Here's how the part is built. I have some questions about the finished solid (model axes, mm). Face numbers are marked on the shaded views. A direction names the side the tool comes from. Give positions to 0.01 mm unless a question says otherwise; leave off trailing zeros. Write each loop counter-clockwise with the first axis right and the second up, starting at its lowest first coordinate (ties: lowest second). Pieces come first, ordered by that corner, then holes. Notation, with made-up numbers: (40.5, 18.25) -> (75.5, 18.25) arc R27 ccw to (75.5, 45.25) -> close; hole circle Ø11 at (-24, -10). An arc over 180 degrees is marked (long way). Use one line per item in the form item = value.
```python
from build123d import *

# Parameters (mm, degrees)
SKETCH_1_W          = 8
SKETCH_1_H          = 48.14748393
SKETCH_1_R          = 1.65
EXTRUDE_1_DEPTH     = 53
EXTRUDE_1_2_DEPTH   = 53
SKETCH_2_W          = 20
SKETCH_2_H          = 3
EXTRUDE_2_DEPTH     = 80
SKETCH_3_R          = 14.5
SKETCH_3_R_2        = 2.25
CUT_EXTRUDE_1_DEPTH = 20
SKETCH_4_W          = 48.14748393
SKETCH_4_H          = 36
CUT_EXTRUDE_2_DEPTH = 15
SKETCH_6_W          = 8
SKETCH_6_H          = 15
CUT_EXTRUDE_4_DEPTH = 6


with BuildPart() as part:
    # Sketch 1 → Extrude 1 (new body)
    with BuildSketch(Plane(origin=(0, 0, 0), x_dir=(1, 0, 0), z_dir=(0, 1, 0))):
        with Locations((44, 0)):
            Rectangle(SKETCH_1_W, SKETCH_1_H)
        with Locations(Location((44, 0, 0), (0, 0, 90))):
            Circle(SKETCH_1_R, mode=Mode.SUBTRACT)
        with Locations(Location((44, -12, 0), (0, 0, 90))):
            Circle(SKETCH_1_R, mode=Mode.SUBTRACT)
        with Locations(Location((44, 12, 0), (0, 0, 270))):
            Circle(SKETCH_1_R, mode=Mode.SUBTRACT)
    extrude(amount=EXTRUDE_1_DEPTH)



with BuildPart() as body_2:
    # Sketch 1 → Extrude 1 2 (new body)
    with BuildSketch(Plane(origin=(0, 0, 0), x_dir=(1, 0, 0), z_dir=(0, 1, 0))):
        with Locations((-44, 0)):
            Rectangle(SKETCH_1_W, SKETCH_1_H)
        with Locations(Location((-44, 0, 0), (0, 0, 270))):
            Circle(SKETCH_1_R, mode=Mode.SUBTRACT)
        with Locations(Location((-44, -12, 0), (0, 0, 270))):
            Circle(SKETCH_1_R, mode=Mode.SUBTRACT)
        with Locations(Location((-44, 12, 0), (0, 0, 90))):
            Circle(SKETCH_1_R, mode=Mode.SUBTRACT)
    extrude(amount=EXTRUDE_1_2_DEPTH)


with BuildPart() as part_1:
    add(part.part)

    add(body_2.part)  # Extrude 2 merges body 2
    # Sketch 2 → Extrude 2 (add)
    with BuildSketch(Plane(origin=(-40, 0, 0), x_dir=(0, 0, -1), z_dir=(1, 0, 0))):
        with Locations((0, 1.5)):
            Rectangle(SKETCH_2_W, SKETCH_2_H)
    extrude(amount=EXTRUDE_2_DEPTH)

    # Sketch 3 → Cut-Extrude 1 (cut)
    with BuildSketch(Plane(origin=(48, 0, 0), x_dir=(0, 0, -1), z_dir=(1, 0, 0))):
        with Locations((-19.073741965, 30)):
            Circle(SKETCH_3_R)
        with Locations((-19.073741965, 47.5)):
            Circle(SKETCH_3_R_2)
        with Locations((-18.617981623, 12.505935792)):
            Circle(SKETCH_3_R_2)
    extrude(amount=-CUT_EXTRUDE_1_DEPTH, mode=Mode.SUBTRACT)

    # Sketch 4 → Cut-Extrude 2 (cut)
    with BuildSketch(Plane.ZY.offset(48)):
        with Locations((0, 35)):
            Rectangle(SKETCH_4_W, SKETCH_4_H)
    extrude(amount=-CUT_EXTRUDE_2_DEPTH, mode=Mode.SUBTRACT)

    # Sketch 6 → Cut-Extrude 4 (cut)
    with BuildSketch(Plane(origin=(0, 17, 0), x_dir=(1, 0, 0), z_dir=(0, 1, 0))):
        with Locations((-44, 0)):
            Rectangle(SKETCH_6_W, SKETCH_6_H)
    extrude(amount=-CUT_EXTRUDE_4_DEPTH, mode=Mode.SUBTRACT)


solid = part_1.part
```
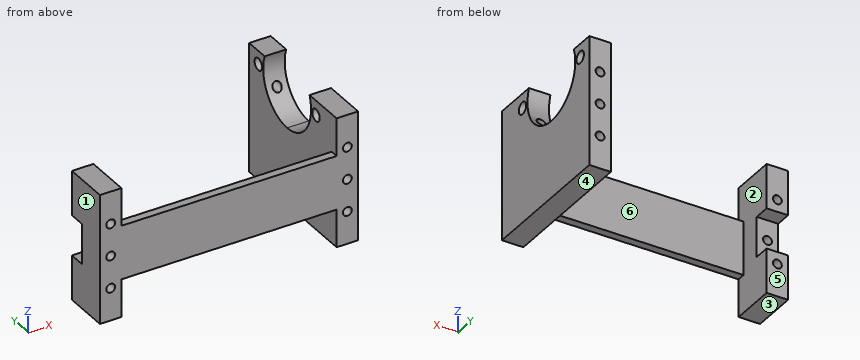
Q1. I want a section at C-C, the plane z = -12. Write out the boundary of the cut face in (x, y).
Result set:
outline = (-48, 0) -> (-45.65, 0) -> (-45.65, 17) -> (-48, 17) -> close; (-42.35, 0) -> (-40, 0) -> (-40, 17) -> (-42.35, 17) -> close; (40, 0) -> (42.35, 0) -> (42.35, 53) -> (40, 53) -> close; (45.65, 0) -> (48, 0) -> (48, 53) -> (45.65, 53) -> close
Q2. If I drill on line 1 along Z through (x, y) = (-44, 7.5); line 2 along X through (y, z) = (7.5, -12); line 3 along X through (y, z) = (3.5, -18), over which ranges is the centre line in solid material (lowest first)? Write a range as from..to.
Result set:
line_1 = -24.07..-13.65, -10.35..-1.65, 1.65..10.35, 13.65..24.07
line_2 = -48..-45.65, -42.35..-40, 40..42.35, 45.65..48
line_3 = -48..-40, 40..48
Q3. Which directions (+Z, -Z, +X, -X, +Y, -Y) give clear straight access to the entire face, cutting with the end or side of a thin tool? Please do the marked faces 4, 5 and 6.
Result set:
face_4 = -Z, +X, -X, +Y, -Y
face_5 = +Z, -Z, -X, +Y
face_6 = +Z, -Z, +Y
Q4. I want a section at B-B, the plane x = -44. Write out the boundary of the cut face in (y, z).
Result set:
outline = (0, -24.07) -> (17, -24.07) -> (17, -13.65) -> (0, -13.65) -> close; (0, -10.35) -> (17, -10.35) -> (17, -7.5) -> (11, -7.5) -> (11, -1.65) -> (0, -1.65) -> close; (0, 1.65) -> (11, 1.65) -> (11, 7.5) -> (17, 7.5) -> (17, 10.35) -> (0, 10.35) -> close; (0, 13.65) -> (17, 13.65) -> (17, 24.07) -> (0, 24.07) -> close
Q5. Will these pins go through, and if not, where does the flat tip stop? pin 1 Ø3 at (x, z) = (-44, 12) entering from -Y; pin 2 Ø14.5 at (y, z) = (35.5, 0) entering from -X; pin 3 Ø2.5 at (x, y) = (-4, 2) entering from -Z; pin 4 Ø4 at (x, z) = (-46, -17) entering from +Y.
Result set:
pin_1 = through
pin_2 = 40
pin_3 = -10
pin_4 = 17
Q6. I want a section at D-D, the plane y = 47.5. Write out the boundary of the cut face in (x, z).
Result set:
outline = (40, -24.07) -> (48, -24.07) -> (48, 16.82) -> (40, 16.82) -> close; (40, 21.32) -> (48, 21.32) -> (48, 24.07) -> (40, 24.07) -> close; hole circle Ø3.3 at (44, -12); hole circle Ø3.3 at (44, 0); hole circle Ø3.3 at (44, 12)
Q7. If we mould it in two halves opening along X, with no side actions, what happens to the marked faces 1, 2 and 3? For each: +X half, -X half, draft (parallel to the pull), parting line (faces both ways), or undercut.
Result set:
face_1 = -X half
face_2 = undercut
face_3 = draft
Q8. I want a section at A-A, the plane y = 5.5. Write out the boundary of the cut face in (x, z), and give its area (3 significant figures).
Result set:
outline = (-48, -24.07) -> (-40, -24.07) -> (-40, 24.07) -> (-48, 24.07) -> close; (40, -24.07) -> (48, -24.07) -> (48, 24.07) -> (40, 24.07) -> close; hole circle Ø3.3 at (-44, -12); hole circle Ø3.3 at (-44, 0); hole circle Ø3.3 at (-44, 12); hole circle Ø3.3 at (44, -12); hole circle Ø3.3 at (44, 0); hole circle Ø3.3 at (44, 12)
area = 719 mm2
